```python
from build123d import *

# Parameters (mm, degrees)
DODANIE_WYCI_GNI_CIE1_DEPTH = 1
SZKIC2_R                    = 0.5
SZKIC2_R_2                  = 1
WYTNIJ_WYCI_GNI_CIE1_DEPTH  = 1
ZAOKR_GLENIE1_R             = 1
SZKIC3_W                    = 1
SZKIC3_H                    = 1
WYTNIJ_WYCI_GNI_CIE2_DEPTH  = 10


with BuildPart() as part:
    # Szkic1 → Dodanie-wyciągnięcie1 (new body)
    with BuildSketch(Plane(origin=(0, 0, 0), x_dir=(1, 0, 0), z_dir=(0, 1, 0))):
        Polygon((0, 0), (17.8, 0), (17.8, 10.2), (3.2, 10.2), (3.2, 9.2), (1, 9.2), (1, 5), (0, 5), align=None)
    extrude(amount=DODANIE_WYCI_GNI_CIE1_DEPTH)

    # Szkic2 → Wytnij-wyciągnięcie1 (cut)
    with BuildSketch(Plane(origin=(0, 1, 0), x_dir=(1, 0, 0), z_dir=(0, 1, 0))):
        with Locations(Location((12.2, 9.3, 0), (0, 0, 270))):
            Circle(SZKIC2_R)
        with Locations(Location((16.2, 9.3, 0), (0, 0, 270))):
            Circle(SZKIC2_R)
        with Locations(Location((6.3, 1.95, 0), (0, 0, 270))):
            Circle(SZKIC2_R_2)
        with Locations(Location((13.65, 1.95, 0), (0, 0, 270))):
            Circle(SZKIC2_R_2)
    extrude(amount=-WYTNIJ_WYCI_GNI_CIE1_DEPTH, mode=Mode.SUBTRACT)

    # Zaokrąglenie1
    zaokr_glenie1_edges = [part.edges().sort_by_distance(p)[0] for p in [
        (0, 0.5, 0),
    ]]
    fillet(zaokr_glenie1_edges, radius=ZAOKR_GLENIE1_R)

    # Szkic3 → Wytnij-wyciągnięcie2 (cut)
    with BuildSketch(Plane(origin=(0, 1, 0), x_dir=(1, 0, 0), z_dir=(0, 1, 0))):
        with Locations((3.7, 9.7)):
            Rectangle(SZKIC3_W, SZKIC3_H)
    extrude(amount=-WYTNIJ_WYCI_GNI_CIE2_DEPTH, mode=Mode.SUBTRACT)


solid = part.part
```
The model under review builds one solid part; all positions refer to its coordinate system, in mm. A direction names the side the tool comes from. Give positions to 0.01 mm unless a question says otherwise; leave off trailing zeros. Write each loop counter-clockwise with the first axis right and the second up, starting at its lowest first coordinate (ties: lowest second). Pieces come first, ordered by that corner, then holes.
(1) Consider section D-D, the plane x = 6.5. Give the boundary of the cut face in (y, z), and give its area (3 significant figures).
(2) The part is to be moulded in two halves that separate along X. For faces 3 (the cylindrical face through (12.696, 0.507, -9.365)), 4 (the flat face through (17.8, 0.5, -5)), 5 (the flat face through (0, 0.5, -3)), say which applies: released by +X, released by -X, zero draft, split by the parting line, or undercut.
(3) Consider section A-A, the plane x = 12.2. Give the boundary of the cut face in (y, z), and give its area (3 significant figures).
(4) Tool access review of faces 1 (the flat face through (1, 0.5, -7.1)), 2 (the flat face through (11.1, 0.5, -10.2)): name each direction out of +Z, -Z, +X, -X, +Y, -Y from which nothing blocks a thin tool from reaching the whole face with its end or side.
(5) Consider section B-B, the plane y = 0.15. Give the boundary of the cut face in (x, z).
(6) Consider section C-C, the plane z = -1.95. Give the boundary of the cut face in (x, y), and give its area (3 significant figures).
(7) To check wall thickness, follow L1, parallel to X at y = 0.35, z = -9.3; L2, parallel to X at y = 0.2, z = -1.95; L3, parallel to Z at x = 3.25, y = 0.8. State the ranges of each line that lie inside material, in increasing order.
Returned:
1. outline: (0, -10.2) - (1, -10.2) - (1, -2.93) - (0, -2.93) - close; (0, -0.97) - (1, -0.97) - (1, 0) - (0, 0) - close
1. area: 8.24 mm2
2. face 3: undercut
2. face 4: released by +X
2. face 5: released by -X
3. outline: (0, -10.2) - (1, -10.2) - (1, -9.8) - (0, -9.8) - close; (0, -8.8) - (1, -8.8) - (1, 0) - (0, 0) - close
3. area: 9.20 mm2
4. face 1: -Z, -X, +Y, -Y
4. face 2: -Z, +X, -X, +Y, -Y
5. outline: (0, -5) - (1, -5) - (1, -9.2) - (4.2, -9.2) - (4.2, -10.2) - (17.8, -10.2) - (17.8, 0) - (1, 0) arc R1 ccw to (0, -1) - close; hole circle Ø2 at (6.3, -1.95); hole circle Ø1 at (12.2, -9.3); hole circle Ø2 at (13.65, -1.95); hole circle Ø1 at (16.2, -9.3)
6. outline: (0, 0) - (5.3, 0) - (5.3, 1) - (0, 1) - close; (7.3, 0) - (12.65, 0) - (12.65, 1) - (7.3, 1) - close; (14.65, 0) - (17.8, 0) - (17.8, 1) - (14.65, 1) - close
6. area: 13.8 mm2
7. L1: x = 4.2 to 11.7, 12.7 to 15.7, 16.7 to 17.8
7. L2: x = 0 to 5.3, 7.3 to 12.65, 14.65 to 17.8
7. L3: z = -9.2 to 0
